```python
from build123d import *

# Parameters (mm, degrees)
SKETCH_1_W               = 80
SKETCH_1_H               = 40
EXTRUDE_1_DEPTH          = 2
SKETCH_2_R               = 3
EXTRUDE_2_DEPTH          = 6
SKETCH_3_R               = 1.5
CUT_EXTRUDE_1_DEPTH      = 1
CUT_EXTRUDE_1_DEPTH_BACK = 9
SKETCH_4_R               = 2
CUT_EXTRUDE_2_DEPTH      = 7
CUT_EXTRUDE_2_DEPTH_BACK = 3
FILLET_1_R               = 2
FILLET_2_R               = 2
FILLET_3_R               = 2
FILLET_4_R               = 2


with BuildPart() as part:
    # Эскиз1 → Бобышка-Вытянуть1 (new body)
    with BuildSketch(Plane(origin=(0, 0, 0), x_dir=(1, 0, 0), z_dir=(0, 1, 0))):
        with Locations((40, -20)):
            Rectangle(SKETCH_1_W, SKETCH_1_H)
    extrude(amount=EXTRUDE_1_DEPTH)

    # Эскиз2 → Бобышка-Вытянуть2 (add)
    with BuildSketch(Plane(origin=(0, 2, 0), x_dir=(1, 0, 0), z_dir=(0, 1, 0))):
        with Locations((10.6, -6.6)):
            Circle(SKETCH_2_R)
        with Locations((10.6, -33.4)):
            Circle(SKETCH_2_R)
        with Locations((69.4, -6.6)):
            Circle(SKETCH_2_R)
        with Locations((69.4, -33.4)):
            Circle(SKETCH_2_R)
    extrude(amount=EXTRUDE_2_DEPTH)

    # Эскиз3 → Вырез-Вытянуть1 (cut, two sides)
    with BuildSketch(Plane(origin=(0, 8, 0), x_dir=(1, 0, 0), z_dir=(0, 1, 0))) as cut_extrude_1_sk:
        with Locations((10.6, -6.6)):
            Circle(SKETCH_3_R)
        with Locations((10.6, -33.4)):
            Circle(SKETCH_3_R)
        with Locations((69.4, -6.6)):
            Circle(SKETCH_3_R)
        with Locations((69.4, -33.4)):
            Circle(SKETCH_3_R)
    extrude(amount=CUT_EXTRUDE_1_DEPTH, mode=Mode.SUBTRACT)
    extrude(cut_extrude_1_sk.sketch, amount=-CUT_EXTRUDE_1_DEPTH_BACK, mode=Mode.SUBTRACT)

    # Эскиз4 → Вырез-Вытянуть2 (cut, two sides)
    with BuildSketch(Plane(origin=(0, 2, 0), x_dir=(1, 0, 0), z_dir=(0, 1, 0))) as cut_extrude_2_sk:
        with Locations((4, -20)):
            Circle(SKETCH_4_R)
        with Locations((76, -20)):
            Circle(SKETCH_4_R)
    extrude(amount=CUT_EXTRUDE_2_DEPTH, mode=Mode.SUBTRACT)
    extrude(cut_extrude_2_sk.sketch, amount=-CUT_EXTRUDE_2_DEPTH_BACK, mode=Mode.SUBTRACT)

    # Скругление1
    fillet_1_edges = [part.edges().sort_by_distance(p)[0] for p in [
        (0, 1, 0),
    ]]
    fillet(fillet_1_edges, radius=FILLET_1_R)

    # Скругление2
    fillet_2_edges = [part.edges().sort_by_distance(p)[0] for p in [
        (0, 1, 40),
    ]]
    fillet(fillet_2_edges, radius=FILLET_2_R)

    # Скругление3
    fillet_3_edges = [part.edges().sort_by_distance(p)[0] for p in [
        (80, 1, 40),
    ]]
    fillet(fillet_3_edges, radius=FILLET_3_R)

    # Скругление4
    fillet_4_edges = [part.edges().sort_by_distance(p)[0] for p in [
        (80, 1, 0),
    ]]
    fillet(fillet_4_edges, radius=FILLET_4_R)


solid = part.part
```
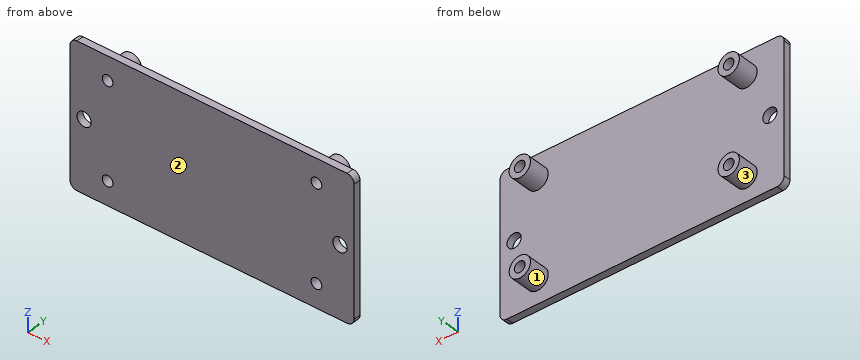
Check sheet for the modelled part. Datum: model origin and axes. Units: mm. Face numbers are marked on the shaded views. Coordinates: 2 decimals unless noted, no trailing zeros. Loops run counter-clockwise (first coordinate to the right, second up) from the corner with the lowest first, then second, coordinate; pieces in that order, holes last. Notation, with made-up numbers: M 10.5,-23 L 24.5,-23 A23 cw 24.5,12 Z; hole C 76,-38.5 d6. An arc over 180 degrees is marked long. Answer as a JSON object with one key per item and string values.
1. Sectioned sample at A-A on y = 4. Record the cut outline in (x, z), and give its area (3 significant figures).
Outcome:
{"outline": "C 10.6,6.6 d6; C 10.6,33.4 d6; C 69.4,6.6 d6; C 69.4,33.4 d6; hole C 10.6,6.6 d3; hole C 10.6,33.4 d3; hole C 69.4,6.6 d3; hole C 69.4,33.4 d3", "area": "84.8 mm²"}
2. Sectioned sample at C-C on z = 20. Record the cut outline in (x, y).
Outcome:
{"outline": "M 0,0 L 2,0 L 2,2 L 0,2 Z; M 6,0 L 74,0 L 74,2 L 6,2 Z; M 78,0 L 80,0 L 80,2 L 78,2 Z"}
3. Depth check by flat-ended pin: P1, Ø4, axis at x = 66, y = 5.5, coming from the +Z side; P2, Ø4.5, axis at x = 4, z = 20, coming from the +Y side. Enter the tip coordinate at first touch or a pass-through.
Outcome:
{"P1": "z = 36.05", "P2": "y = 2"}
4. Sectioned sample at D-D on x = 10.6. Record the cut outline in (y, z).
Outcome:
{"outline": "M 0,0 L 2,0 L 2,3.6 L 8,3.6 L 8,5.1 L 0,5.1 Z; M 0,8.1 L 8,8.1 L 8,9.6 L 2,9.6 L 2,30.4 L 8,30.4 L 8,31.9 L 0,31.9 Z; M 0,34.9 L 8,34.9 L 8,36.4 L 2,36.4 L 2,40 L 0,40 Z"}
5. Sectioned sample at B-B on x = 76. Record the cut outline in (y, z), and give its area (3 significant figures).
Outcome:
{"outline": "M 0,0 L 2,0 L 2,18 L 0,18 Z; M 0,22 L 2,22 L 2,40 L 0,40 Z", "area": "72.0 mm²"}
6. Release check for a two-part mould opening along X. For the marked faces 1, 2 and 3 record: pulls with the +X half, pulls with the -X half, needs draft (parallel to the pull), parting line crosses it, or undercut.
Outcome:
{"face 1": "undercut", "face 2": "needs draft", "face 3": "undercut"}
7. Scan lines: L1, parallel to X at y = 0.55, z = 20; L2, parallel to X at y = 6, z = 6.6; L3, parallel to Z at x = 10.6, y = 2.5. Record each from-to range of solid material in increasing order. Write a range as from..to.
Outcome:
{"L1": "0..2, 6..74, 78..80", "L2": "7.6..9.1, 12.1..13.6, 66.4..67.9, 70.9..72.4", "L3": "3.6..5.1, 8.1..9.6, 30.4..31.9, 34.9..36.4"}
